For this review, take the finished solid that the model builds, in its own axes (mm). A direction names the side the tool comes from. Give positions to 0.01 mm unless a question says otherwise; leave off trailing zeros. Loops run counter-clockwise (first coordinate to the right, second up) from the corner with the lowest first, then second, coordinate; pieces in that order, holes last. Notation, with made-up numbers: M 10,1.25 L 51,1.25 A8 ccw 51,7.25 Z; hole C 55.25,12.5 d9. An arc over 180 degrees is marked long. Use CSV: the item, a comma, the result in double quotes. Start each with the question number.
1. Take a section at C-C, the plane z = -83.5. Write out the cut boundary in (x, y), and give its area (3 significant figures).
2. Take a section at A-A, the plane z = -18. Write out the cut boundary in (x, y), and give its area (3 significant figures).
3. Tool access review of faces 1 (the face through (3.772, -9.986, -59.135)), 2 (the face through (0, 2.358, -6)), 3 (the face through (-15, 7, -23)): name each direction out of +Z, -Z, +X, -X, +Y, -Y from which nothing blocks a thin tool from reaching the whole face with its end or side.
4. Take a section at D-D, the plane z = -6.5. Write out the cut boundary in (x, y).
5. Take a section at B-B, the plane y = 12.5. Write out the cut boundary in (x, z).
6. Insertion check: P1, Ø5, axis at x = -13, y = 13, coming from the +Z side; P2, Ø11, axis at x = -8, y = 1, coming from the +Z side; P3, Ø12, axis at x = 10.5, z = -35, coming from the +Y side; P4, Ø6, axis at y = 21.5, z = -21.5, coming from the +X side. Each pin has a flat end and moves straight along its axis. Give the tip position at first contact, or say it passes through.
7. To check wall thickness, follow line 1 (Y direction, x = 0, z = -22.35); line 2 (Z direction, x = -10, y = 20); line 3 (Z direction, x = -10, y = 2). State the ranges of each line that lie inside material, in increasing order. Write a range as [from, to].
8. The part is to be moulded in two halves that separate along Y. For faces 4 (the face through (0, 0, 0)), 5 (the face through (-9.139, 21.334, -82.292)), 6 (the face through (8, 20, -23)), say which applies: pulls with the +Y half, pulls with the -Y half, needs draft (parallel to the pull), parting line crosses it, or undercut.
from build123d import *

# Parameters (mm, degrees)
SKETCH1_R           = 3
BOSS_EXTRUDE1_DEPTH = 16
CUT_EXTRUDE1_DEPTH  = 13
SKETCH4_R           = 6
BOSS_EXTRUDE2_DEPTH = 6
SKETCH5_R           = 18.4
BOSS_EXTRUDE3_DEPTH = 22
SKETCH6_R           = 17.4
BOSS_EXTRUDE4_DEPTH = 30.7
SKETCH7_R           = 17
BOSS_EXTRUDE5_DEPTH = 15.4
SKETCH8_R           = 2
SKETCH8_R_2         = 1.5
CUT_EXTRUDE2_DEPTH  = 1
CUT_EXTRUDE3_DEPTH  = 1
CUT_EXTRUDE4_DEPTH  = 0.5


with BuildPart() as part:
    # Sketch1 → Boss-Extrude1 (new body)
    with BuildSketch(Plane.XY):
        Circle(SKETCH1_R)
    extrude(amount=-BOSS_EXTRUDE1_DEPTH)

    # Sketch2 → Cut-Extrude1 (cut)
    with BuildSketch(Plane.XY):
        with BuildLine():
            Line((-1.854051563, 2.358493757), (1.854051563, 2.358493757))
            ThreePointArc((1.854051563, 2.358493757), (0, 3), (-1.854051563, 2.358493757))
        make_face()
    extrude(amount=-CUT_EXTRUDE1_DEPTH, mode=Mode.SUBTRACT)

    # Sketch4 → Boss-Extrude2 (add)
    with BuildSketch(Plane(origin=(0, 0, -16), x_dir=(-1, 0, 0), z_dir=(0, 0, -1))):
        Circle(SKETCH4_R)
    extrude(amount=BOSS_EXTRUDE2_DEPTH)

    # Sketch5 → Boss-Extrude3 (add)
    with BuildSketch(Plane(origin=(0, 0, -22), x_dir=(-1, 0, 0), z_dir=(0, 0, -1))):
        with Locations((0, 7)):
            Circle(SKETCH5_R)
    extrude(amount=BOSS_EXTRUDE3_DEPTH)

    # Sketch6 → Boss-Extrude4 (add)
    with BuildSketch(Plane(origin=(0, 0, -44), x_dir=(-1, 0, 0), z_dir=(0, 0, -1))):
        with Locations((0, 7)):
            Circle(SKETCH6_R)
    extrude(amount=BOSS_EXTRUDE4_DEPTH)

    # Sketch7 → Boss-Extrude5 (add)
    with BuildSketch(Plane(origin=(0, 0, -74.7), x_dir=(-1, 0, 0), z_dir=(0, 0, -1))):
        with Locations((0, 7)):
            Circle(SKETCH7_R)
    extrude(amount=BOSS_EXTRUDE5_DEPTH)

    # Sketch8 → Cut-Extrude2 (cut)
    with BuildSketch(Plane.XY.offset(-22)):
        with Locations((0, 22.4)):
            Circle(SKETCH8_R)
        with Locations((13.336791218, -0.7)):
            Circle(SKETCH8_R)
        with Locations((-13.336791218, -0.7)):
            Circle(SKETCH8_R)
        with Locations((-15.4, 7)):
            Circle(SKETCH8_R_2)
        with Locations((-7.65, 20.423393759)):
            Circle(SKETCH8_R_2)
        with Locations((7.85, 20.423393759)):
            Circle(SKETCH8_R_2)
        with Locations((15.6, 7)):
            Circle(SKETCH8_R_2)
        with Locations((7.85, -6.423393759)):
            Circle(SKETCH8_R_2)
        with Locations((-7.65, -6.423393759)):
            Circle(SKETCH8_R_2)
    extrude(amount=-CUT_EXTRUDE2_DEPTH, mode=Mode.SUBTRACT)

    # Sketch9 → Cut-Extrude3 (cut)
    with BuildSketch(Plane.XY.offset(-22)):
        with BuildLine():
            ThreePointArc((7.451414877, -2.911428571), (0, 8), (-7.451414877, -2.911428571))
            ThreePointArc((-7.451414877, -2.911428571), (0, 19.4), (7.451414877, -2.911428571))
        make_face()
    extrude(amount=-CUT_EXTRUDE3_DEPTH, mode=Mode.SUBTRACT)

    # Sketch10 → Cut-Extrude4 (cut)
    with BuildSketch(Plane.XY.offset(-23)):
        Polygon((0.198821757, 22.604844617), (1.765091395, 22.604844617), (1.765091395, 22.195155383), (0.198821757, 22.195155383), (0.198821757, 20.628885745), (-0.210867478, 20.628885745), (-0.210867478, 22.195155383), (-1.777137116, 22.195155383), (-1.777137116, 22.604844617), (-0.210867478, 22.604844617), (-0.210867478, 24.171114255), (0.198821757, 24.171114255), align=None)
        Polygon((13.414780982, -0.974607001), (12.631646163, -2.331036297), (12.276844878, -2.126191679), (13.059979697, -0.769762384), (11.703550402, 0.013372435), (11.908395019, 0.36817372), (13.264824315, -0.414961099), (14.047959134, 0.941468197), (14.402760419, 0.736623579), (13.6196256, -0.619805716), (14.976054895, -1.402940535), (14.771210278, -1.75774182), align=None)
        Polygon((-13.613602739, -0.630237616), (-14.396737558, 0.726191679), (-14.041936273, 0.931036297), (-13.258801454, -0.425392999), (-11.902372159, 0.35774182), (-11.697527541, 0.002940535), (-13.053956837, -0.780194284), (-12.270822018, -2.136623579), (-12.625623303, -2.341468197), (-13.408758122, -0.985038901), (-14.765187417, -1.76817372), (-14.970032035, -1.413372435), align=None)
    extrude(amount=-CUT_EXTRUDE4_DEPTH, mode=Mode.SUBTRACT)


solid = part.part
Result set:
1,outline,"C 0,7 d34"
1,area,"908 mm2"
2,outline,"C 0,0 d12"
2,area,"113 mm2"
3,face 1,"-Z"
3,face 2,"+Z, +X, -X, +Y"
3,face 3,"+Z"
4,outline,"M -1.85,2.36 A3 ccw long 1.85,2.36 Z"
5,outline,"M -17.56,-44 L -16.51,-44 L -16.51,-74.7 L -16.09,-74.7 L -16.09,-90.1 L 16.09,-90.1 L 16.09,-74.7 L 16.51,-74.7 L 16.51,-44 L 17.56,-44 L 17.56,-22 L 11.11,-22 L 11.11,-23 L -11.11,-23 L -11.11,-22 L -17.56,-22 Z"
6,P1,"z = -22"
6,P2,"z = 0"
6,P3,"y = 24.84"
6,P4,"x = 14.33"
7,line 1,"[-11.4, 8], [19.4, 20.4], [24.4, 25.4]"
7,line 2,"[-90.1, -22]"
7,line 3,"[-90.1, -23]"
8,face 4,"needs draft"
8,face 5,"parting line crosses it"
8,face 6,"undercut"
